Read the model definition and answer for the solid it produces. Units are mm, in the model's axes. Face numbers are marked on the shaded views. A direction names the side the tool comes from. Give positions to 0.01 mm unless a question says otherwise; leave off trailing zeros. Loops run counter-clockwise (first coordinate to the right, second up) from the corner with the lowest first, then second, coordinate; pieces in that order, holes last. Notation, with made-up numbers: M 36,-15 L 73,-15 A26 ccw 73,5 Z; hole C -5,33 d1. An arc over 180 degrees is marked long. Return JSON: item names as keys, results as strings. Group by question number.
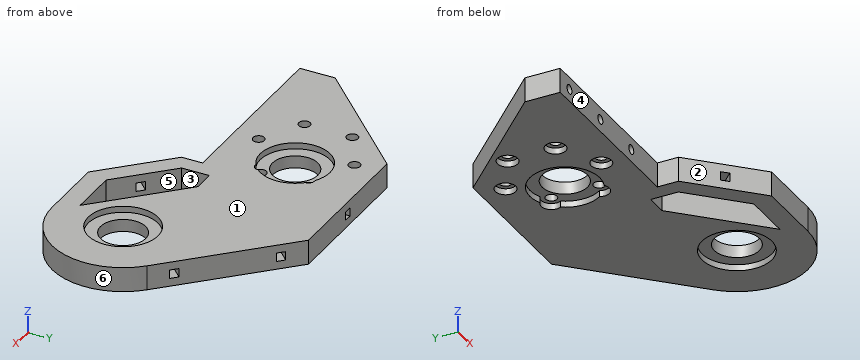
```python
from build123d import *

# Parameters (mm, degrees)
MODEL_R                  = 7.35
MODEL_R_2                = 7.3
MODEL_R_3                = 1.85
RESSALTO_EXTRUS_O1_DEPTH = 8
ESBO_O3_R                = 11.3
CORTE_EXTRUS_O1_DEPTH    = 2
ESBO_O4_R                = 11.3
CORTE_EXTRUS_O2_DEPTH    = 2
ESBO_O2_R                = 3.3
CORTE_EXTRUS_O4_DEPTH    = 2
ESBO_O7_W                = 2.8
ESBO_O7_H                = 2.8
CORTE_EXTRUS_O6_DEPTH    = 6
ESBO_O8_W                = 2.8
ESBO_O8_H                = 2.8
CORTE_EXTRUS_O7_DEPTH    = 6
ESBO_O10_W               = 2.8
ESBO_O10_H               = 2.8
CORTE_EXTRUS_O9_DEPTH    = 6
RESSALTO_EXTRUS_O3_DEPTH = 8
ESBO_O6_R                = 1.5
CORTE_EXTRUS_O5_DEPTH    = 10
ESBO_O15_R               = 11.3
RESSALTO_EXTRUS_O4_DEPTH = 8


with BuildPart() as part:
    # Model → Ressalto-extrusão1 (new body)
    with BuildSketch(Plane.XY):
        with BuildLine():
            Line((0, 0), (39, 0))
            Line((39, 0), (39.7, 0))
            Line((39.7, 0), (39.7, -6.854833996))
            Line((39.7, -6.854833996), (52.445166004, -19.6))
            Line((52.445166004, -19.6), (59.445166004, -26.6))
            Line((59.445166004, -26.6), (81.699998871, -26.6))
            ThreePointArc((81.699998871, -26.6), (102.949229032, -12.401719466), (97.963455967, 12.663455967))
            Line((97.963455967, 12.663455967), (63.677897161, 46.949014774))
            Line((63.677897161, 46.949014774), (50.111140335, 46.949014774))
            Line((50.111140335, 46.949014774), (15.50707852, 46.949014774))
            Line((15.50707852, 46.949014774), (0, 31.441936254))
            Line((0, 31.441936254), (0, 0))
        make_face()
        with Locations((59.072583002, 19.027416998)):
            Circle(MODEL_R, mode=Mode.SUBTRACT)
        with Locations((81.7, -3.6)):
            Circle(MODEL_R_2, mode=Mode.SUBTRACT)
        with Locations((6.960594046, 15.730973227)):
            Circle(MODEL_R_3, mode=Mode.SUBTRACT)
        with Locations((6.960594046, 31.230973227)):
            Circle(MODEL_R_3, mode=Mode.SUBTRACT)
        with Locations((20.383987804, 38.980973227)):
            Circle(MODEL_R_3, mode=Mode.SUBTRACT)
        with Locations((33.807381563, 31.230973227)):
            Circle(MODEL_R_3, mode=Mode.SUBTRACT)
        with Locations((33.807381563, 15.730973227)):
            Circle(MODEL_R_3, mode=Mode.SUBTRACT)
        with Locations((20.383987804, 7.980973227)):
            Circle(MODEL_R_3, mode=Mode.SUBTRACT)
        with Locations((27.383987804, 23.480973227)):
            Circle(MODEL_R, mode=Mode.SUBTRACT)
        Polygon((72, -15), (52, 5), (45, 5), (45, -4), (61, -20), (77, -20), align=None, mode=Mode.SUBTRACT)
    extrude(amount=RESSALTO_EXTRUS_O1_DEPTH)

    # Esboço3 → Corte-extrusão1 (cut)
    with BuildSketch(Plane.XY):
        with Locations((81.7, -3.6)):
            Circle(ESBO_O3_R)
        with Locations((59.0726, 19.0274)):
            Circle(ESBO_O3_R)
        with Locations((27.384004802, 23.480956229)):
            Circle(ESBO_O3_R)
    extrude(amount=CORTE_EXTRUS_O1_DEPTH, mode=Mode.SUBTRACT)

    # Esboço4 → Corte-extrusão2 (cut)
    with BuildSketch(Plane.XY.offset(8)):
        with Locations((81.7, -3.6)):
            Circle(ESBO_O4_R)
        with Locations((59.0726, 19.0274)):
            Circle(ESBO_O4_R)
        with Locations((27.384004802, 23.480956229)):
            Circle(ESBO_O4_R)
    extrude(amount=-CORTE_EXTRUS_O2_DEPTH, mode=Mode.SUBTRACT)

    # Esboço2 → Corte-extrusão4 (cut)
    with BuildSketch(Plane.XY):
        with Locations((6.960594802, 15.730956229)):
            Circle(ESBO_O2_R)
        with Locations((6.960594802, 31.230956229)):
            Circle(ESBO_O2_R)
        with Locations((33.807404802, 15.730956229)):
            Circle(ESBO_O2_R)
        with Locations((20.384004802, 38.980956229)):
            Circle(ESBO_O2_R)
        with Locations((33.807404802, 31.230956229)):
            Circle(ESBO_O2_R)
        with Locations((20.384004802, 7.980976229)):
            Circle(ESBO_O2_R)
    extrude(amount=CORTE_EXTRUS_O4_DEPTH, mode=Mode.SUBTRACT)

    # Esboço7 → Corte-extrusão6 (cut)
    with BuildSketch(Plane(origin=(55.313455967, 55.313455967, 0), x_dir=(0, 0, -1), z_dir=(0.707106781, 0.707106781, 0))):
        with Locations((-4, -52.072657306)):
            Rectangle(ESBO_O7_W, ESBO_O7_H)
        with Locations((-4, -20.072657306)):
            Rectangle(ESBO_O7_W, ESBO_O7_H)
    extrude(amount=-CORTE_EXTRUS_O6_DEPTH, mode=Mode.SUBTRACT)

    # Esboço8 → Corte-extrusão7 (cut)
    with BuildSketch(Plane(origin=(0, 46.949014774, 0), x_dir=(1, 0, 0), z_dir=(0, 1, 0))):
        with Locations((39.59248784, -4)):
            Rectangle(ESBO_O8_W, ESBO_O8_H)
    extrude(amount=-CORTE_EXTRUS_O7_DEPTH, mode=Mode.SUBTRACT)

    # Esboço10 → Corte-extrusão9 (cut)
    with BuildSketch(Plane(origin=(16.422583002, 16.422583002, 0), x_dir=(0, 0, 1), z_dir=(-0.707106781, -0.707106781, 0))):
        with Locations((4, -46.881179593)):
            Rectangle(ESBO_O10_W, ESBO_O10_H)
    extrude(amount=-CORTE_EXTRUS_O9_DEPTH, mode=Mode.SUBTRACT)

    # Esboço13 → Ressalto-extrusão3 (add)
    with BuildSketch(Plane.XY.offset(8)):
        Polygon((0, 31.441936254), (-20, 11.441936254), (-20, 0), (0, 0), align=None)
    extrude(amount=-RESSALTO_EXTRUS_O3_DEPTH)

    # Esboço6 → Corte-extrusão5 (cut)
    with BuildSketch(Plane.XZ):
        with Locations((4.7, 4)):
            Circle(ESBO_O6_R)
        with Locations((23.7, 4)):
            Circle(ESBO_O6_R)
        with Locations((-14.3, 4)):
            Circle(ESBO_O6_R)
    extrude(amount=-CORTE_EXTRUS_O5_DEPTH, mode=Mode.SUBTRACT)

    # Esboço15 → Ressalto-extrusão4 (add)
    with BuildSketch(Plane.XY.offset(8)):
        with Locations((59.0726, 19.0274)):
            Circle(ESBO_O15_R)
    extrude(amount=-RESSALTO_EXTRUS_O4_DEPTH)


solid = part.part
```
1. Straight lines are drawn through the part: line 1 along X through (y, z) = (-7.5, 5.25); line 2 along Y through (x, z) = (10, 1.5); line 3 along Y through (x, z) = (32.5, 4.25). For each, find the intervals that lie inside material, in ascending order.
2. Flat-ended cylindrical pins translate along their axes: P1, Ø3.5, axis at x = 23.7, z = 4, coming from the -Y side; P2, Ø1.8, axis at x = 4.7, z = 4, coming from the -Y side; P3, Ø1.5, axis at x = 83.5, z = 2.5, coming from the -Y side. Find the tip coordinate at first contact, or state that the pin passes through.
3. Find section A-A (x = 85). Write down the section's boundary in (y, z), and give its area (3 significant figures).
4. For the marked faces 4, 5 and 6, determine the directions among +Z, -Z, +X, -X, +Y, -Y from which every point of the face is accessible in a straight line to the end or side of a thin tool.
5. Find section B-B (x = 7.5). Write down the section's boundary in (y, z), and give its area (3 significant figures).
6. The mould has two halves that part along Y. Classify the marked faces 1, 2 and 3: +Y half, -Y half, draft (parallel to the pull), parting line (faces both ways), or undercut.
7. Find section C-C (x = -14.3). Write down the section's boundary in (y, z).
Result:
{
 "1": {"line 1": "x = 40.35 to 48.5, 64.5 to 75.53, 87.87 to 104.37", "line 2": "y = 0 to 14.45, 17.02 to 29.95, 32.52 to 41.44", "line 3": "y = 0 to 14.42, 17.04 to 18.2, 28.76 to 29.92, 32.54 to 46.95"},
 "2": {"P1": "stops at y = 0", "P2": "stops at y = 10", "P3": "stops at y = -26.58"},
 "3": {"outline": "M -26.36,0 L -14.41,0 L -14.41,2 L -10.11,2 L -10.11,6 L -14.41,6 L -14.41,8 L -26.36,8 Z; M 2.91,2 L 7.21,2 L 7.21,0 L 25.63,0 L 25.63,8 L 7.21,8 L 7.21,6 L 2.91,6 Z", "area": "277 mm2"},
 "4": {"face 4": "+Z, -Z, -X, -Y", "face 5": "+Z, -Z", "face 6": "+Z, -Z, +X"},
 "5": {"outline": "M 0,0 L 12.48,0 L 12.48,2 L 13.96,2 L 13.96,8 L 0,8 Z; M 17.5,2 L 18.99,2 L 18.99,0 L 27.98,0 L 27.98,2 L 29.46,2 L 29.46,8 L 17.5,8 Z; M 33,2 L 34.49,2 L 34.49,0 L 38.94,0 L 38.94,8 L 33,8 Z", "area": "243 mm2"},
 "6": {"face 1": "draft", "face 2": "-Y half", "face 3": "undercut"},
 "7": {"outline": "M 0,0 L 17.14,0 L 17.14,8 L 0,8 L 0,5.5 L 10,5.5 L 10,2.5 L 0,2.5 Z"}
}
